For this review, take the finished solid that the model builds, in its own axes (mm). A direction names the side the tool comes from. Coordinates: 2 decimals unless noted, no trailing zeros. Loops run counter-clockwise (first coordinate to the right, second up) from the corner with the lowest first, then second, coordinate; pieces in that order, holes last.
```python
from build123d import *

# Parameters (mm, degrees)
SKETCH2_R           = 1.5
SKETCH5_R           = 1.5
SKETCH1_R           = 1.5
BOSS_EXTRUDE1_DEPTH = 5


with BuildPart() as part:
    # Sweep1: sweep along a path in Sketch3
    with BuildLine(Plane(origin=(0, 0, 0), x_dir=(-0.8090169943749461, 0, 0.5877852522924749), z_dir=(-0.5877852522924749, 0, -0.8090169943749461))) as sweep1_path:
        Line((4, 0), (4, 2.5))
        Line((4, 2.5), (0, 2.5))
    # Sketch2 → Sweep1 (sweep)
    with BuildSketch(Plane(origin=(0, 0, 0), x_dir=(1, 0, 0), z_dir=(0, 1, 0))):
        with Locations((-3.236067977, -2.351141009)):
            Circle(SKETCH2_R)
    sweep(path=sweep1_path.line, transition=Transition.RIGHT)

    # Sweep2: sweep along a path in Sketch6
    with BuildLine(Plane(origin=(0, 0, 0), x_dir=(0.8090169943749507, 0, 0.5877852522924687), z_dir=(-0.5877852522924687, 0, 0.8090169943749507))) as sweep2_path:
        Line((4, 0), (4, 2.5))
        Line((4, 2.5), (0, 2.5))
    # Sketch5 → Sweep2 (sweep)
    with BuildSketch(Plane(origin=(0, 0, 0), x_dir=(1, 0, 0), z_dir=(0, 1, 0))):
        with Locations((3.236067977, -2.351141009)):
            Circle(SKETCH5_R)
    sweep(path=sweep2_path.line, transition=Transition.RIGHT)

    # Sketch1 → Boss-Extrude1 (add)
    with BuildSketch(Plane(origin=(0, 0, 0), x_dir=(1, 0, 0), z_dir=(0, 1, 0))):
        with Locations(Location((0, 0, 0), (0, 0, 270))):
            Circle(SKETCH1_R)
    extrude(amount=BOSS_EXTRUDE1_DEPTH)


solid = part.part
```
Q1. Wall thickness on probe 1 along X at (y, z) = (0.5, 3.4); probe 2 along X at (y, z) = (3.65, 2.95); probe 3 along Y at (x, z) = (3, 2.1): over which ranges is each line inside the solid? List them lowest first.
Q2. The part is to be moulded in two halves that separate along X. For faces 3 (the face through (3, 0, 2)), 4 (the face through (4.62, 1.58, 2.93)), 5 (the face through (-4.4, 1.6, 3.3)), say which applies: +X half, -X half, draft (parallel to the pull), parting line (faces both ways), or undercut.
Q3. Consider section A-A (y = 3.9). State the section outline as (x, z) points, then the cut area to 3 significant figures.
Q4. Machinability: for faces 1 (the face through (0.07, 2.46, -1.5)), 2 (the face through (0, 5, 0)), which of the approach directions +Z, -Z, +X, -X, +Y, -Y give a long, thin tool a straight path to every point of the face, cutting with its end or side? Answer none if there is none.
Q5. For pin 1 Ø3 at (x, y) = (2.5, 4) entering from -Z; pin 2 Ø2 at (x, z) = (2.5, 1) entering from +Y; pin 3 Ø1.5 at (x, y) = (-0.5, 3) entering from +Z, all flat-tipped, find the tip position at first contact; note any pin that passes through.
Model answer:
1. probe 1: x = -4.31 to -2.16, 2.16 to 4.31
1. probe 2: x = -4.61 to -2.42, 2.42 to 4.61
1. probe 3: y = 0 to 4
2. face 3: draft
2. face 4: undercut
2. face 5: undercut
3. outline: (-4.69, 2.74) - (-1.45, 0.39) arc R1.5 ccw (long way) to (1.45, 0.39) - (4.69, 2.74) arc R1.5 ccw to (4.05, 3.61) - (0.82, 1.26) arc R1.5 ccw to (-0.82, 1.26) - (-4.05, 3.61) arc R1.5 ccw to start
3. area: 15.7 mm2
4. face 1: none
4. face 2: +Z, -Z, +X, -X, +Y
5. pin 1: stops at z = -1.12
5. pin 2: stops at y = 4
5. pin 3: stops at z = 2.71
